```python
from build123d import *

# Parameters (mm, degrees)
CYLINDER001_R     = 3
CYLINDER001_DEPTH = 8
PAD007_DEPTH      = 3
CYLINDER002_R     = 3
CYLINDER002_DEPTH = 8
SKETCH029_R       = 1.5
POCKET021_DEPTH   = 10
CHAMFER018_SIZE   = 1
SKETCH030_R       = 1.75
POCKET022_DEPTH   = 5
CHAMFER019_SIZE   = 0.5


with BuildPart() as keypadbracketscrewcylinder:
    # Cylinder001 → Cylinder001 (new body)
    with BuildSketch(Plane(origin=(25.4, 13.5, 18), x_dir=(1, 0, 0), z_dir=(0, 0, 1))):
        Circle(CYLINDER001_R)
    extrude(amount=CYLINDER001_DEPTH)


with BuildPart() as keypadbracketpad007:
    # Sketch028 → Pad007 (new body)
    with BuildSketch(Plane.XY.offset(18)):
        with BuildLine():
            Line((0, -3.5), (10, -3.5))
            Line((10, -3.5), (10, 10.5))
            Line((10, 10.5), (25.4, 10.5))
            ThreePointArc((25.4, 10.5), (28.354423, 12.979055), (26.42606, 16.319078))
            Line((26.42606, 16.319078), (5, 24.117526))
            Line((5, 24.117526), (5, 46.062474))
            Line((5, 46.062474), (26.42606, 53.860922))
            ThreePointArc((26.42606, 53.860922), (28.354423, 57.200945), (25.4, 59.68))
            Line((25.4, 59.68), (0, 59.68))
            Line((0, 59.68), (0, -3.5))
        make_face()
    extrude(amount=PAD007_DEPTH)


with BuildPart() as keypadbracketscrewholeschamfer018:
    # Cylinder002 → Cylinder002 (new body)
    with BuildSketch(Plane(origin=(25.4, 56.68, 18), x_dir=(1, 0, 0), z_dir=(0, 0, 1))):
        Circle(CYLINDER002_R)
    extrude(amount=CYLINDER002_DEPTH)

    # Fusion003: union KeypadBracketScrewCylinder, KeypadBracketPad007
    add(keypadbracketscrewcylinder.part)
    add(keypadbracketpad007.part)

    # Sketch029 → Pocket021 (cut)
    with BuildSketch(Plane.XY.offset(26)):
        with Locations((25.4, 13.5)):
            Circle(SKETCH029_R)
        with Locations((25.4, 56.68)):
            Circle(SKETCH029_R)
    extrude(amount=-POCKET021_DEPTH, mode=Mode.SUBTRACT)

    # Chamfer018
    chamfer018_edges = [keypadbracketscrewholeschamfer018.edges().sort_by_distance(p)[0] for p in [
        (23.9, 56.68, 26),
        (23.9, 13.5, 26),
    ]]
    chamfer(chamfer018_edges, length=CHAMFER018_SIZE)


with BuildPart() as keypadbracketprintingchamfer019_final:
    # Part__Mirroring004: instance of KeypadBracketScrewHolesChamfer018
    add(keypadbracketscrewholeschamfer018.part.mirror(Plane(origin=(0, 0, 0), x_dir=(0, -1, 0), z_dir=(1, 0, 0))))

    # Fusion004: union KeypadBracketScrewHolesChamfer018
    add(keypadbracketscrewholeschamfer018.part)

    # Sketch030 → Pocket022 (cut)
    with BuildSketch(Plane.XY.offset(21)):
        with Locations((0, 0.5)):
            Circle(SKETCH030_R)
        with Locations((0, 55.5)):
            Circle(SKETCH030_R)
    extrude(amount=-POCKET022_DEPTH, mode=Mode.SUBTRACT)

    # Chamfer019
    chamfer019_edges = [keypadbracketprintingchamfer019_final.edges().sort_by_distance(p)[0] for p in [
        (-25.4, 15, 18),
        (-25.4, 12, 18),
        (0, 57.25, 18),
        (0, 53.75, 18),
        (0, 2.25, 18),
        (0, -1.25, 18),
        (-27.52132, 58.80132, 18),
        (-27.857456, 54.959271, 18),
        (0, 59.68, 18),
        (-15.71303, 49.961698, 18),
        (27.52132, 58.80132, 18),
        (-5, 35.09, 18),
        (27.857456, 54.959271, 18),
        (-15.71303, 20.218302, 18),
        (15.71303, 49.961698, 18),
        (-27.857456, 15.220729, 18),
        (5, 35.09, 18),
        (-27.52132, 11.37868, 18),
        (15.71303, 20.218302, 18),
        (-17.7, 10.5, 18),
        (27.857456, 15.220729, 18),
        (-10, 3.5, 18),
        (27.52132, 11.37868, 18),
        (0, -3.5, 18),
        (17.7, 10.5, 18),
        (10, 3.5, 18),
        (25.4, 58.18, 18),
        (25.4, 55.18, 18),
        (25.4, 15, 18),
        (25.4, 12, 18),
        (-25.4, 58.18, 18),
        (-25.4, 55.18, 18),
    ]]
    chamfer(chamfer019_edges, length=CHAMFER019_SIZE)


solid = keypadbracketprintingchamfer019_final.part
```
Can you work these out from the model? Positions are in its coordinate system, mm. A direction names the side the tool comes from. Coordinates: 2 decimals unless noted, no trailing zeros. Loops run counter-clockwise (first coordinate to the right, second up) from the corner with the lowest first, then second, coordinate; pieces in that order, holes last. Notation, with made-up numbers: M 13,11 L 46,11 A12 cw 46,24 Z; hole C 65,29 d6. An arc over 180 degrees is marked long. Put each result on its own line as item: value. Start each with the question number.
(1) Which directions (+Z, -Z, +X, -X, +Y, -Y) give clear straight access to the entire face, cutting with the end or side of a thin tool? Please do faces 5 (the face through (15.563, 49.907, 19.732)), 6 (the face through (-15.31, 50.08, 18.25)), 7 (the face through (18, 10.5, 20)), 8 (the face through (27.99, 57.19, 18.14)), 9 (the face through (0, 59.68, 20)).
(2) We'd pull the mould along X, two halves only. Please class faces 1 (the face through (26.83, 13.95, 21.8)), 2 (the face through (0, -3.5, 20)), 3 (the face through (28.26, 14.4, 23.03)), 4 (the face through (-10, 3, 20)): +X half, -X half, draft (parallel to the pull), parting line (faces both ways), or undercut.
(3) Imagine slicing it at D-D on z = 19.75. List the corners of the cut face in (x, y) for me, and give its area (3 significant figures).
(4) Imagine slicing it at C-C on x = 0. List the corners of the cut face in (y, z) for me, and give its area (3 significant figures).
(5) Imagine slicing it at A-A on z = 24. List the corners of the cut face in (x, y) for me, and give its area (3 significant figures).
(6) Will these pins go through, and if not, where does the flat tip stop? pin 1 Ø0.8 at (y, z) = (34.5, 19.5) entering from -X; pin 2 Ø1.5 at (x, y) = (-1.5, 45) entering from +Z; pin 3 Ø4 at (x, z) = (-21.5, 21) entering from -Y; pin 4 Ø3 at (y, z) = (50.5, 24.5) entering from +X.
(7) I need wall thicknesses on probe 1 along Y at (x, z) = (25.4, 21.75); probe 2 along Y at (x, z) = (-25.5, 19.25); probe 3 along Z at (x, y) = (-10.5, 18). Which ranges of each line are inside material? Lowest first, please.
(8) Imagine slicing it at B-B on y = 13.5. List the corners of the cut face in (x, z) for me.
Worked answers:
1. face 5: +Z, -Z, +X
1. face 6: -Z, -X
1. face 7: +Z, -Z, +X, -Y
1. face 8: -Z, +X
1. face 9: +Z, -Z, +X, -X, +Y
2. face 1: undercut
2. face 2: draft
2. face 3: undercut
2. face 4: -X half
3. outline: M -26.43,16.32 A3 ccw -25.4,10.5 L -10,10.5 L -10,-3.5 L 10,-3.5 L 10,10.5 L 25.4,10.5 A3 ccw 26.43,16.32 L 5,24.12 L 5,46.06 L 26.43,53.86 A3 ccw 25.4,59.68 L -25.4,59.68 A3 ccw -26.43,53.86 L -5,46.06 L -5,24.12 Z; hole C -25.4,13.5 d3; hole C -25.4,56.68 d3; hole C 0,0.5 d3.5; hole C 0,55.5 d3.5; hole C 25.4,13.5 d3; hole C 25.4,56.68 d3
3. area: 1,590 mm2
4. outline: M -3.5,18.5 L -3,18 L -1.75,18 L -1.25,18.5 L -1.25,21 L -3.5,21 Z; M 2.25,18.5 L 2.75,18 L 53.25,18 L 53.75,18.5 L 53.75,21 L 2.25,21 Z; M 57.25,18.5 L 57.75,18 L 59.18,18 L 59.68,18.5 L 59.68,21 L 57.25,21 Z
4. area: 168 mm2
5. outline: C -25.4,13.5 d6; C -25.4,56.68 d6; C 25.4,13.5 d6; C 25.4,56.68 d6; hole C -25.4,13.5 d3; hole C -25.4,56.68 d3; hole C 25.4,13.5 d3; hole C 25.4,56.68 d3
5. area: 84.8 mm2
6. pin 1: stops at x = -5
6. pin 2: stops at z = 21
6. pin 3: stops at y = 10.5
6. pin 4: passes through
7. probe 1: y = 10.5 to 12, 15 to 16.5, 53.68 to 55.18, 58.18 to 59.68
7. probe 2: y = 10.5 to 12, 15 to 16.66, 53.52 to 55.18, 58.18 to 59.68
7. probe 3: z = 18 to 21
8. outline: M -28.4,18.5 L -27.9,18 L -27.4,18 L -26.9,18.5 L -26.9,25 L -27.9,26 L -28.4,26 Z; M -23.9,18.5 L -23.4,18 L 23.4,18 L 23.9,18.5 L 23.9,25 L 22.9,26 L 22.4,26 L 22.4,21 L -22.4,21 L -22.4,26 L -22.9,26 L -23.9,25 Z; M 26.9,18.5 L 27.4,18 L 27.9,18 L 28.4,18.5 L 28.4,26 L 27.9,26 L 26.9,25 Z
